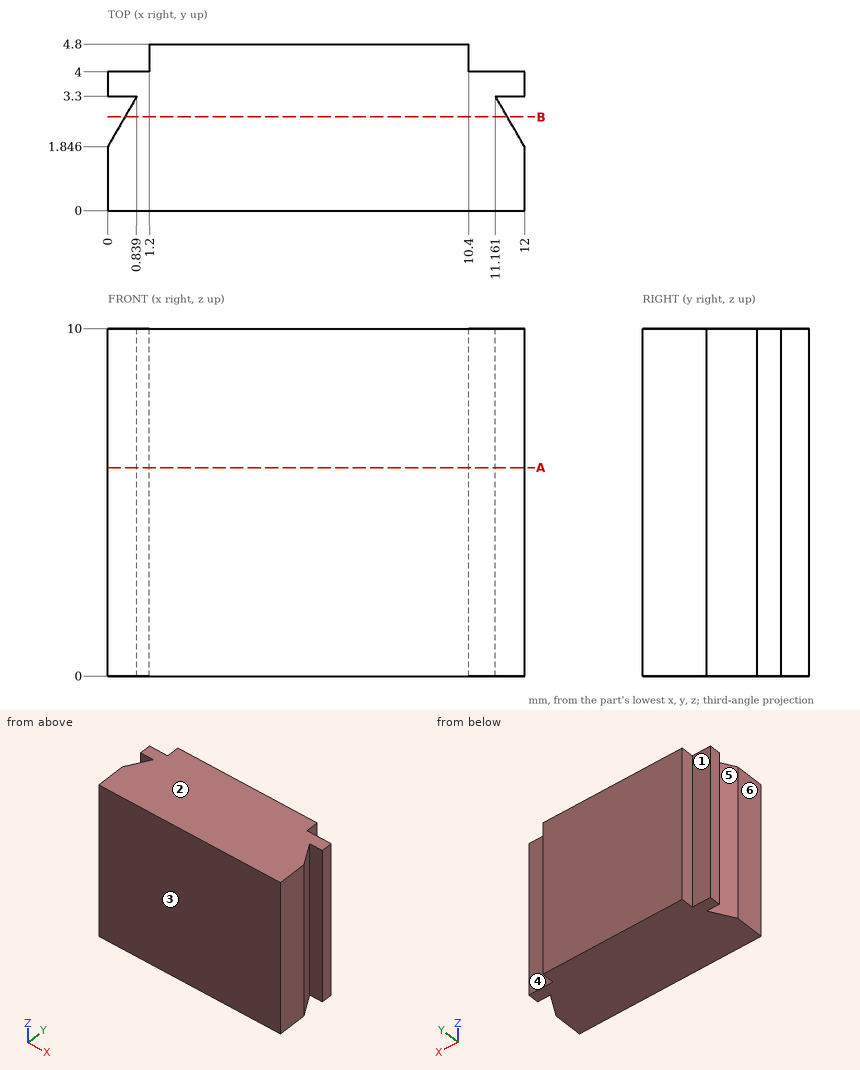
The drawing under review shows one solid part. Ordinate dimensions are in mm from its lowest x, y, z. A direction names the side the tool comes from. Give positions to 0.01 mm unless a question says otherwise; leave off trailing zeros. Write each loop counter-clockwise with the first axis right and the second up, starting at its lowest first coordinate (ties: lowest second). Pieces come first, ordered by that corner, then holes. Notation, with made-up numbers: M 30,0.25 L 75,0.25 A27 cw 75,34.25 Z; hole C -39.75,-18.5 d10. An arc over 180 degrees is marked long. Write each question's results on one line, items separated by ' | '. Start each with the question number.
1. Mouldability with a two-part tool opening along Y and no side actions: class the marked faces 3, 4, 5 and 6 as released by +Y, released by -Y, zero draft, split by the parting line, or undercut.
2. For probe 1 along Y at (x, z) = (1, 1.5); probe 2 along X at (y, z) = (4.5, 8.75); probe 3 along Y at (x, z) = (0.75, 7.25) (1 decimal), list the stretches that pass through material, from the lowest coordinate up. Write a range as [from, to].
3. We need section B-B (y = 2.7). Write out the cut boundary in (x, z), and give its area (3 significant figures).
4. We need section A-A (z = 6). Write out the cut boundary in (x, y).
5. For the marked faces 1 and 2, list the 3-axis set-ups (+Z, -Z, +X, -X, +Y, -Y) from which the entire face can be reached by the end or side of a thin tool; tool diameter is ignored.
6. Insertion check: pin 1 Ø0.6 at (y, z) = (4.5, 4.5) entering from +X; pin 2 Ø1.8 at (x, z) = (11.5, 7) entering from +Y. Each pin has a flat end and moves straight along its axis. Give the tip position at first contact, or say it passes through.
Results found:
1) face 3: released by -Y | face 4: released by +Y | face 5: undercut | face 6: zero draft
2) probe 1: y = [0, 4] | probe 2: x = [1.2, 10.4] | probe 3: y = [0, 3.1], [3.3, 4]
3) outline: M 0.49,0 L 11.51,0 L 11.51,10 L 0.49,10 Z | area: 110 mm^2
4) outline: M 0,0 L 12,0 L 12,1.85 L 11.16,3.3 L 12,3.3 L 12,4 L 10.4,4 L 10.4,4.8 L 1.2,4.8 L 1.2,4 L 0,4 L 0,3.3 L 0.84,3.3 L 0,1.85 Z
5) face 1: +Z, -Z, -X, +Y | face 2: +Z, +X, -X, +Y, -Y
6) pin 1: stops at x = 10.4 | pin 2: stops at y = 4
